Source: CAD feature listing. Evaluate the final solid. Frame: model axes, mm. Give positions to 0.01 mm unless a question says otherwise; leave off trailing zeros. Order: outer loops, then holes, each group sorted by start corner. A loop starts at its lowest first (then second) coordinate and runs counter-clockwise, first axis right, second up. Notation, with made-up numbers: (50.25, 88) - (69.25, 88) arc R23 ccw to (69.25, 100) - close; hole circle Ø11 at (-20.5, 65). An arc over 180 degrees is marked (long way). Answer as CSV lines item,"result".
```python
from build123d import *

# Parameters (mm, degrees)
F0_R          = 18.2753
F0_R_2        = 16.2687
F1_DEPTH      = 27.178
F2_R          = 1.5875
F3_DEPTH      = 18.2763
F3_DEPTH_BACK = 18.2763
F4_R          = 1.5875
F5_DEPTH      = 18.2763001
F5_DEPTH_BACK = 18.2763001


with BuildPart() as f1:
    # F0 (on Right) → F1 (new body, symmetric)
    with BuildSketch(Plane.YZ):
        Circle(F0_R)
        Circle(F0_R_2, mode=Mode.SUBTRACT)
    extrude(amount=F1_DEPTH, both=True)

    # F2 (on Top) → F3 (cut, two sides)
    with BuildSketch(Plane.XY) as f3_sk:
        Circle(F2_R)
    extrude(amount=-F3_DEPTH, mode=Mode.SUBTRACT)
    extrude(f3_sk.sketch, amount=F3_DEPTH_BACK, mode=Mode.SUBTRACT)

    # F4 (on Front) → F5 (cut, two sides)
    with BuildSketch(Plane.XZ) as f5_sk:
        with Locations((-7.493, 0)):
            Circle(F4_R)
        with Locations((7.493, 0)):
            Circle(F4_R)
    extrude(amount=-F5_DEPTH, mode=Mode.SUBTRACT)
    extrude(f5_sk.sketch, amount=F5_DEPTH_BACK, mode=Mode.SUBTRACT)


solid = f1.part
```
(1) Contact query for flat-ended pins moving along their axis: pin 1 (1.9 mm diameter, centred on x = 7.493, z = 0, fed in from +Y); pin 2 (12 mm diameter, centred on x = 19.5, y = 9, fed in from +Z); pin 3 (6 mm diameter, centred on x = 20.5, y = 4.5, fed in from +Z); pin 4 (10 mm diameter, centred on x = -18.5, y = 11, fed in from +Z). Output: stop coordinate, or through.
Completed:
pin 1,"through"
pin 2,"z = 18.03"
pin 3,"z = 18.21"
pin 4,"z = 17.26"
(2) Cut plane C-C (z = 7.5). Return loops of the section in (x, y), then the cut area to 3 significant figures.
Completed:
outline,"(-27.18, -16.67) - (27.18, -16.67) - (27.18, -14.44) - (-27.18, -14.44) - close; (-27.18, 14.44) - (27.18, 14.44) - (27.18, 16.67) - (-27.18, 16.67) - close"
area,"242 mm²"
(3) Cut plane A-A (z = 0). Return loops of the section in (x, y), then the cut area to 3 significant figures.
Completed:
outline,"(-27.18, -18.28) - (-9.08, -18.28) - (-9.08, -16.27) - (-27.18, -16.27) - close; (-27.18, 16.27) - (-9.08, 16.27) - (-9.08, 18.28) - (-27.18, 18.28) - close; (-5.91, -18.28) - (5.91, -18.28) - (5.91, -16.27) - (-5.91, -16.27) - close; (-5.91, 16.27) - (5.91, 16.27) - (5.91, 18.28) - (-5.91, 18.28) - close; (9.08, -18.28) - (27.18, -18.28) - (27.18, -16.27) - (9.08, -16.27) - close; (9.08, 16.27) - (27.18, 16.27) - (27.18, 18.28) - (9.08, 18.28) - close"
area,"193 mm²"
(4) Ray query, line 1 (Z direction, x = -5, y = 0); line 2 (Z direction, x = 14, y = 8); line 3 (Y direction, x = -24, z = -15). Return the intervals inside material, ascending. Write a range as from..to.
Completed:
line 1,"-18.28..-16.27, 16.27..18.28"
line 2,"-16.43..-14.17, 14.17..16.43"
line 3,"-10.44..-6.3, 6.3..10.44"
(5) Cut plane B-B (y = 0). Return loops of the section in (x, z), then the cut area to 3 significant figures.
Completed:
outline,"(-27.18, -18.28) - (-1.59, -18.28) - (-1.59, -16.27) - (-27.18, -16.27) - close; (-27.18, 16.27) - (-1.59, 16.27) - (-1.59, 18.28) - (-27.18, 18.28) - close; (1.59, -18.28) - (27.18, -18.28) - (27.18, -16.27) - (1.59, -16.27) - close; (1.59, 16.27) - (27.18, 16.27) - (27.18, 18.28) - (1.59, 18.28) - close"
area,"205 mm²"
(6) Cut plane D-D (x = 0). Return loops of the section in (y, z), then the cut area to 3 significant figures.
Completed:
outline,"(-1.59, -18.21) - (-1.59, -16.19) arc R16.27 cw to (-1.59, 16.19) - (-1.59, 18.21) arc R18.28 ccw to start; (1.59, -18.21) arc R18.28 ccw to (1.59, 18.21) - (1.59, 16.19) arc R16.27 cw to (1.59, -16.19) - close"
area,"205 mm²"
(7) Mould query, pull axis X, two halves, no side actions, for faces 1 (the cylindrical face through (5.907, -17.219, 0.07)), 2 (the flat face through (-27.178, -15, -7)), 3 (the flat face through (27.178, -15, -7)). Classes: released by +X, released by -X, zero draft, split by the parting line, or undercut.
Completed:
face 1,"undercut"
face 2,"released by -X"
face 3,"released by +X"
